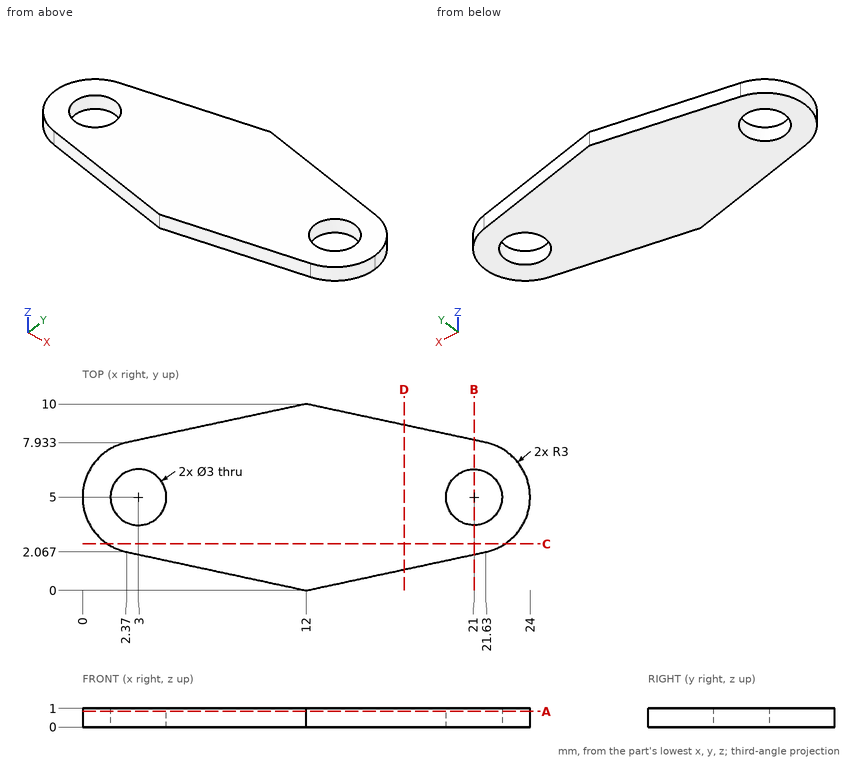
Job drawing, mm, ordinate dimensions from the low corner. One solid piece. Coordinates: 2 decimals unless noted, no trailing zeros. Write each loop counter-clockwise with the first axis right and the second up, starting at its lowest first coordinate (ties: lowest second). Pieces come first, ordered by that corner, then holes. Notation, with made-up numbers: (-38, 49) -> (18, 49) arc R30 ccw to (18, 86) -> close; hole circle Ø4 at (-3, 15). An arc over 180 degrees is marked (long way). Use CSV: the item, a comma, the result in double quotes. Start each with the question number.
Item 1: Band-saw the part on A-A, the plane z = 0.85. Write the cut outline in (x, y).
Item 2: Band-saw the part on D-D, the plane x = 17.25. Write the cut outline in (y, z).
Item 3: Band-saw the part on B-B, the plane x = 21. Write the cut outline in (y, z).
Item 4: Band-saw the part on C-C, the plane y = 2.5. Write the cut outline in (x, z).
Item 5: Wall check: probe 1 along Y at (x, z) = (21, 0.4); probe 2 along Y at (x, z) = (20, 0.65) (1 decimal); probe 3 along Y at (x, z) = (8.5, 0.4). Give the ranges that are in metal, low to high.
Response values:
1,outline,"(2.37, 2.07) -> (12, 0) -> (21.63, 2.07) arc R3 ccw to (24, 5) arc R3 ccw to (21.63, 7.93) -> (12, 10) -> (2.37, 7.93) arc R3 ccw to start; hole circle Ø3 at (3, 5); hole circle Ø3 at (21, 5)"
2,outline,"(1.13, 0) -> (8.87, 0) -> (8.87, 1) -> (1.13, 1) -> close"
3,outline,"(1.93, 0) -> (3.5, 0) -> (3.5, 1) -> (1.93, 1) -> close; (6.5, 0) -> (8.07, 0) -> (8.07, 1) -> (6.5, 1) -> close"
4,outline,"(1.34, 0) -> (22.66, 0) -> (22.66, 1) -> (1.34, 1) -> close"
5,probe 1,"y = 1.93 to 3.5, 6.5 to 8.07"
5,probe 2,"y = 1.7 to 3.9, 6.1 to 8.3"
5,probe 3,"y = 0.75 to 9.25"
